from build123d import *

# Parameters (mm, degrees)
BOSS_EXTRUDE1_DEPTH = 50.8
CUT_EXTRUDE1_DEPTH  = 2.27


with BuildPart() as part:
    # Sketch2 → Boss-Extrude1 (new body, symmetric)
    with BuildSketch(Plane(origin=(0, 0, 0), x_dir=(1, 0, 0), z_dir=(0, 1, 0))):
        with BuildLine():
            Line((-5.334, 0), (20.066, 0))
            ThreePointArc((20.066, 0), (20.335407684, -0.111592316), (20.447, -0.381))
            Line((20.447, -0.381), (20.447, -0.889))
            ThreePointArc((20.447, -0.889), (20.335407684, -1.158407684), (20.066, -1.27))
            Line((20.066, -1.27), (1.651, -1.27))
            ThreePointArc((1.651, -1.27), (1.381592316, -1.381592316), (1.27, -1.651))
            Line((1.27, -1.651), (1.27, -14.351))
            ThreePointArc((1.27, -14.351), (1.158407684, -14.620407684), (0.889, -14.732))
            Line((0.889, -14.732), (-0.76996875, -14.732))
            ThreePointArc((-0.76996875, -14.732), (-0.904672592, -14.756607134), (-1.021976563, -14.82725))
            ThreePointArc((-1.021976563, -14.82725), (-2.921, -13.97), (-1.021976563, -13.11275))
            ThreePointArc((-1.021976563, -13.11275), (-0.904672592, -13.183392866), (-0.76996875, -13.208))
            Line((-0.76996875, -13.208), (-0.381, -13.208))
            ThreePointArc((-0.381, -13.208), (-0.111592316, -13.096407684), (0, -12.827))
            Line((0, -12.827), (0, -1.651))
            ThreePointArc((0, -1.651), (-0.111592316, -1.381592316), (-0.381, -1.27))
            Line((-0.381, -1.27), (-5.334, -1.27))
            ThreePointArc((-5.334, -1.27), (-5.603407684, -1.158407684), (-5.715, -0.889))
            Line((-5.715, -0.889), (-5.715, -0.381))
            ThreePointArc((-5.715, -0.381), (-5.603407684, -0.111592316), (-5.334, 0))
        make_face()
    extrude(amount=BOSS_EXTRUDE1_DEPTH, both=True)

    # Sketch3 → Cut-Extrude1 (cut, through all)
    with BuildSketch(Plane.XY.offset(1.27)):
        with BuildLine():
            Line((11.71575, 2.38125), (13.30325, 2.38125))
            ThreePointArc((13.30325, 2.38125), (15.6845, 0), (13.30325, -2.38125))
            Line((13.30325, -2.38125), (11.71575, -2.38125))
            ThreePointArc((11.71575, -2.38125), (9.3345, 0), (11.71575, 2.38125))
        make_face()
    extrude(amount=-CUT_EXTRUDE1_DEPTH, mode=Mode.SUBTRACT)


solid = part.part
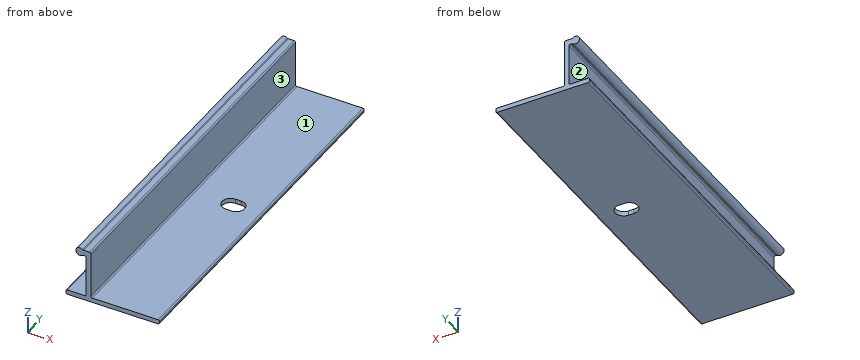
Source: CAD feature listing. Evaluate the final solid. Frame: model axes, mm. Face numbers are marked on the shaded views. Round coordinates to 2 decimals unless told otherwise and drop trailing zeros. Loops run counter-clockwise (first coordinate to the right, second up) from the corner with the lowest first, then second, coordinate; pieces in that order, holes last.
Q1. First-contact query: P1, Ø3.5, axis at y = 14.5, z = 7, coming from the -X side; P2, Ø4, axis at y = -22.5, z = 5, coming from the +X side; P3, Ø1.3, axis at x = 0, y = -14.5, coming from the +Z side. Flat tips, straight axial feed; report the tip coordinate or a pass-through.
Q2. Section C-C, the plane z = 9. Return loops of the section in (x, y), plus the area to 3 significant figures.
Q3. Mould query, pull axis Z, two halves, no side actions, for the marked faces 1, 2 and 3. Classes: pulls with the +Z half, pulls with the -Z half, needs draft (parallel to the pull), parting line crosses it, or undercut.
Q4. Section B-B, the plane y = 31. Return loops of the section in (x, z) (3 decimals), plus the area to 3 significant figures.
Q5. Section D-D, the plane x = 5. Return loops of the section in (y, z).
Q6. Ray query, line 1 (Z direction, x = 4, y = 25); line 2 (X direction, y = 36.5, z = 13.75). Return the intervals inside material, ascending.
Solutions:
1. P1: stops at x = 0
1. P2: stops at x = 1.27
1. P3: stops at z = 14.73
2. outline: (0, -50.8) - (1.27, -50.8) - (1.27, 50.8) - (0, 50.8) - close
2. area: 129 mm2
3. face 1: pulls with the +Z half
3. face 2: undercut
3. face 3: needs draft
4. outline: (-5.715, 0.381) arc R0.381 ccw to (-5.334, 0) - (20.066, 0) arc R0.381 ccw to (20.447, 0.381) - (20.447, 0.889) arc R0.381 ccw to (20.066, 1.27) - (1.651, 1.27) arc R0.381 cw to (1.27, 1.651) - (1.27, 14.351) arc R0.381 ccw to (0.889, 14.732) - (-0.77, 14.732) arc R0.381 cw to (-1.022, 14.827) arc R1.143 ccw (long way) to (-1.022, 13.113) arc R0.381 cw to (-0.77, 13.208) - (-0.381, 13.208) arc R0.381 cw to (0, 12.827) - (0, 1.651) arc R0.381 cw to (-0.381, 1.27) - (-5.334, 1.27) arc R0.381 ccw to (-5.715, 0.889) - close
4. area: 55.5 mm2
5. outline: (-50.8, 0) - (50.8, 0) - (50.8, 1.27) - (-50.8, 1.27) - close
6. line 1: z = 0 to 1.27
6. line 2: x = -2.9 to 1.27
